For this review, take the finished solid that the model builds, in its own axes (mm). A direction names the side the tool comes from. Round coordinates to 2 decimals unless told otherwise and drop trailing zeros. Loops run counter-clockwise (first coordinate to the right, second up) from the corner with the lowest first, then second, coordinate; pieces in that order, holes last. Notation, with made-up numbers: (13, 36) -> (59, 36) arc R28 ccw to (59, 69) -> close; hole circle Ø9 at (-19.5, -29.5). An arc over 180 degrees is marked (long way). Write each question's results on one line, items separated by ' | '.
```python
from build123d import *

# Parameters (mm, degrees)
CROQUIS1_R              = 9.9
SALIENTE_EXTRUIR1_DEPTH = 2.45
CROQUIS2_R              = 4.5
SALIENTE_EXTRUIR2_DEPTH = 4.5
CROQUIS3_R              = 1.5
CROQUIS3_R_2            = 1
CORTAR_EXTRUIR1_DEPTH   = 15.706121175


with BuildPart() as part:
    # Croquis1 → Saliente-Extruir1 (new body)
    with BuildSketch(Plane.XY):
        Circle(CROQUIS1_R)
    extrude(amount=SALIENTE_EXTRUIR1_DEPTH)

    # Croquis2 → Saliente-Extruir2 (add)
    with BuildSketch(Plane.XY.offset(2.45)):
        Circle(CROQUIS2_R)
    extrude(amount=-SALIENTE_EXTRUIR2_DEPTH)

    # Croquis3 → Cortar-Extruir1 (cut, through all)
    with BuildSketch(Plane.XY.offset(2.45)):
        Circle(CROQUIS3_R)
        with Locations((7, 0)):
            Circle(CROQUIS3_R_2)
        with Locations((0, -7)):
            Circle(CROQUIS3_R_2)
        with Locations((-7, 0)):
            Circle(CROQUIS3_R_2)
        with Locations((0, 7)):
            Circle(CROQUIS3_R_2)
    extrude(amount=-CORTAR_EXTRUIR1_DEPTH, mode=Mode.SUBTRACT)


solid = part.part
```
1. Consider section C-C (y = 7). State the section outline as (x, z) points.
Values found:
outline: (-7, 0) -> (-1, 0) -> (-1, 2.45) -> (-7, 2.45) -> close; (1, 0) -> (7, 0) -> (7, 2.45) -> (1, 2.45) -> close
2. For pin 1 (3 mm diameter, centred on x = 7, y = 0, fed in from +Z); pin 2 (2.5 mm diameter, centred on x = 0, y = 7, fed in from -Z); pin 3 (1 mm diameter, centred on x = 7, z = -1.5, fed in from +Y); pin 4 (1.5 mm diameter, centred on y = 5, z = 1, fed in from +X), all flat-tipped, find the tip position at first contact; note any pin that passes through.
Values found:
pin 1: stops at z = 2.45 | pin 2: stops at z = 0 | pin 3: passes through | pin 4: stops at x = 8.94
3. Tool access review of faces 1 (the face through (6.2, -0.6, 1.2)), 2 (the face through (-0.59, 4.46, -1.01)): name each direction out of +Z, -Z, +X, -X, +Y, -Y from which nothing blocks a thin tool from reaching the whole face with its end or side.
Values found:
face 1: +Z, -Z | face 2: -Z
4. Consider section A-A (y = 0). State the section outline as (x, z) points, plus the area to 3 significant figures.
Values found:
outline: (-9.9, 0) -> (-8, 0) -> (-8, 2.45) -> (-9.9, 2.45) -> close; (-6, 0) -> (-4.5, 0) -> (-4.5, -2.05) -> (-1.5, -2.05) -> (-1.5, 2.45) -> (-6, 2.45) -> close; (1.5, -2.05) -> (4.5, -2.05) -> (4.5, 0) -> (6, 0) -> (6, 2.45) -> (1.5, 2.45) -> close; (8, 0) -> (9.9, 0) -> (9.9, 2.45) -> (8, 2.45) -> close | area: 43.7 mm2
5. Consider section B-B (z = 1.85). State the section outline as (x, y) points.
Values found:
outline: circle Ø19.8 at (0, 0); hole circle Ø2 at (-7, 0); hole circle Ø3 at (0, 0); hole circle Ø2 at (0, -7); hole circle Ø2 at (0, 7); hole circle Ø2 at (7, 0)
6. Draft analysis for pull direction X (two halves, no side actions). For faces 3 (the face through (0, -2, -2.05)), 4 (the face through (9.443, 2.974, 1.208)), 5 (the face through (0, -6, 1)), state which applies: released by +X, released by -X, zero draft, split by the parting line, or undercut.
Values found:
face 3: zero draft | face 4: split by the parting line | face 5: undercut
7. To check wall thickness, follow probe 1 along Y at (x, z) = (0, 0.9); probe 2 along Z at (x, y) = (-4.5, 7.5); probe 3 along Y at (x, z) = (-7, 1.45). State the ranges of each line that lie inside material, in increasing order.
Values found:
probe 1: y = -9.9 to -8, -6 to -1.5, 1.5 to 6, 8 to 9.9 | probe 2: z = 0 to 2.45 | probe 3: y = -7 to -1, 1 to 7
